Build history of the part. All positions in model axes, mm. A direction names the side the tool comes from. Give positions to 0.01 mm unless a question says otherwise; leave off trailing zeros. Loops run counter-clockwise (first coordinate to the right, second up) from the corner with the lowest first, then second, coordinate; pieces in that order, holes last. Notation, with made-up numbers: M 67.5,5.25 L 99.5,5.25 A17 ccw 99.5,18.25 Z; hole C 74.25,-19 d11. An arc over 180 degrees is marked long. Answer in a Markdown table with one row per item. Add a question column.
```python
from build123d import *

# Parameters (mm, degrees)
BOSS_EXTRUDE1_DEPTH = 1.5875


with BuildPart() as part:
    # Sketch1 → Boss-Extrude1 (new body)
    with BuildSketch(Plane(origin=(0, 0, 0), x_dir=(1, 0, 0), z_dir=(0, 1, 0))):
        with BuildLine():
            Line((-1.159549536, 2.070936998), (-3.090908521, 3.791368499))
            ThreePointArc((-3.090908521, 3.791368499), (-3.125119474, 3.931396235), (-3.006433754, 4.0132))
            Line((-3.006433754, 4.0132), (-1.7526, 4.0132))
            ThreePointArc((-1.7526, 4.0132), (-1.572994878, 4.087594878), (-1.4986, 4.2672))
            Line((-1.4986, 4.2672), (-1.4986, 4.7498))
            ThreePointArc((-1.4986, 4.7498), (-1.572994878, 4.929405122), (-1.7526, 5.0038))
            Line((-1.7526, 5.0038), (-4.7498, 5.0038))
            ThreePointArc((-4.7498, 5.0038), (-4.929405122, 4.929405122), (-5.0038, 4.7498))
            Line((-5.0038, 4.7498), (-5.0038, 1.7526))
            ThreePointArc((-5.0038, 1.7526), (-4.929405122, 1.572994878), (-4.7498, 1.4986))
            Line((-4.7498, 1.4986), (-4.2672, 1.4986))
            ThreePointArc((-4.2672, 1.4986), (-4.087594878, 1.572994878), (-4.0132, 1.7526))
            Line((-4.0132, 1.7526), (-4.0132, 3.006433754))
            ThreePointArc((-4.0132, 3.006433754), (-3.931396235, 3.125119474), (-3.791368499, 3.090908521))
            Line((-3.791368499, 3.090908521), (-2.070936998, 1.159549536))
            ThreePointArc((-2.070936998, 1.159549536), (-2.023228558, 1.08099247), (-2.0066, 0.9906))
            Line((-2.0066, 0.9906), (-2.0066, 0.7493))
            ThreePointArc((-2.0066, 0.7493), (-1.932205122, 0.569694878), (-1.7526, 0.4953))
            ThreePointArc((-1.7526, 0.4953), (-1.572994878, 0.420905122), (-1.4986, 0.2413))
            Line((-1.4986, 0.2413), (-1.4986, -0.2413))
            ThreePointArc((-1.4986, -0.2413), (-1.572994878, -0.420905122), (-1.7526, -0.4953))
            ThreePointArc((-1.7526, -0.4953), (-1.932205122, -0.569694878), (-2.0066, -0.7493))
            Line((-2.0066, -0.7493), (-2.0066, -0.9906))
            ThreePointArc((-2.0066, -0.9906), (-2.023228558, -1.08099247), (-2.070936998, -1.159549536))
            Line((-2.070936998, -1.159549536), (-3.791368499, -3.090908521))
            ThreePointArc((-3.791368499, -3.090908521), (-3.931396235, -3.125119474), (-4.0132, -3.006433754))
            Line((-4.0132, -3.006433754), (-4.0132, -1.7526))
            ThreePointArc((-4.0132, -1.7526), (-4.087594878, -1.572994878), (-4.2672, -1.4986))
            Line((-4.2672, -1.4986), (-4.7498, -1.4986))
            ThreePointArc((-4.7498, -1.4986), (-4.929405122, -1.572994878), (-5.0038, -1.7526))
            Line((-5.0038, -1.7526), (-5.0038, -4.7498))
            ThreePointArc((-5.0038, -4.7498), (-4.929405122, -4.929405122), (-4.7498, -5.0038))
            Line((-4.7498, -5.0038), (-1.7526, -5.0038))
            ThreePointArc((-1.7526, -5.0038), (-1.572994878, -4.929405122), (-1.4986, -4.7498))
            Line((-1.4986, -4.7498), (-1.4986, -4.2672))
            ThreePointArc((-1.4986, -4.2672), (-1.572994878, -4.087594878), (-1.7526, -4.0132))
            Line((-1.7526, -4.0132), (-3.006433754, -4.0132))
            ThreePointArc((-3.006433754, -4.0132), (-3.125119474, -3.931396235), (-3.090908521, -3.791368499))
            Line((-3.090908521, -3.791368499), (-1.159549536, -2.070936998))
            ThreePointArc((-1.159549536, -2.070936998), (-1.08099247, -2.023228558), (-0.9906, -2.0066))
            Line((-0.9906, -2.0066), (-0.7493, -2.0066))
            ThreePointArc((-0.7493, -2.0066), (-0.569694878, -1.932205122), (-0.4953, -1.7526))
            ThreePointArc((-0.4953, -1.7526), (-0.420905122, -1.572994878), (-0.2413, -1.4986))
            Line((-0.2413, -1.4986), (0.2413, -1.4986))
            ThreePointArc((0.2413, -1.4986), (0.420905122, -1.572994878), (0.4953, -1.7526))
            ThreePointArc((0.4953, -1.7526), (0.569694878, -1.932205122), (0.7493, -2.0066))
            Line((0.7493, -2.0066), (0.9906, -2.0066))
            ThreePointArc((0.9906, -2.0066), (1.08099247, -2.023228558), (1.159549536, -2.070936998))
            Line((1.159549536, -2.070936998), (3.090908521, -3.791368499))
            ThreePointArc((3.090908521, -3.791368499), (3.125119474, -3.931396235), (3.006433754, -4.0132))
            Line((3.006433754, -4.0132), (1.7526, -4.0132))
            ThreePointArc((1.7526, -4.0132), (1.572994878, -4.087594878), (1.4986, -4.2672))
            Line((1.4986, -4.2672), (1.4986, -4.7498))
            ThreePointArc((1.4986, -4.7498), (1.572994878, -4.929405122), (1.7526, -5.0038))
            Line((1.7526, -5.0038), (4.7498, -5.0038))
            ThreePointArc((4.7498, -5.0038), (4.929405122, -4.929405122), (5.0038, -4.7498))
            Line((5.0038, -4.7498), (5.0038, -1.7526))
            ThreePointArc((5.0038, -1.7526), (4.929405122, -1.572994878), (4.7498, -1.4986))
            Line((4.7498, -1.4986), (4.2672, -1.4986))
            ThreePointArc((4.2672, -1.4986), (4.087594878, -1.572994878), (4.0132, -1.7526))
            Line((4.0132, -1.7526), (4.0132, -3.006433754))
            ThreePointArc((4.0132, -3.006433754), (3.931396235, -3.125119474), (3.791368499, -3.090908521))
            Line((3.791368499, -3.090908521), (2.070936998, -1.159549536))
            ThreePointArc((2.070936998, -1.159549536), (2.023228558, -1.08099247), (2.0066, -0.9906))
            Line((2.0066, -0.9906), (2.0066, -0.7493))
            ThreePointArc((2.0066, -0.7493), (1.932205122, -0.569694878), (1.7526, -0.4953))
            ThreePointArc((1.7526, -0.4953), (1.572994878, -0.420905122), (1.4986, -0.2413))
            Line((1.4986, -0.2413), (1.4986, 0.2413))
            ThreePointArc((1.4986, 0.2413), (1.572994878, 0.420905122), (1.7526, 0.4953))
            ThreePointArc((1.7526, 0.4953), (1.932205122, 0.569694878), (2.0066, 0.7493))
            Line((2.0066, 0.7493), (2.0066, 0.9906))
            ThreePointArc((2.0066, 0.9906), (2.023228558, 1.08099247), (2.070936998, 1.159549536))
            Line((2.070936998, 1.159549536), (3.791368499, 3.090908521))
            ThreePointArc((3.791368499, 3.090908521), (3.931396235, 3.125119474), (4.0132, 3.006433754))
            Line((4.0132, 3.006433754), (4.0132, 1.7526))
            ThreePointArc((4.0132, 1.7526), (4.087594878, 1.572994878), (4.2672, 1.4986))
            Line((4.2672, 1.4986), (4.7498, 1.4986))
            ThreePointArc((4.7498, 1.4986), (4.929405122, 1.572994878), (5.0038, 1.7526))
            Line((5.0038, 1.7526), (5.0038, 4.7498))
            ThreePointArc((5.0038, 4.7498), (4.929405122, 4.929405122), (4.7498, 5.0038))
            Line((4.7498, 5.0038), (1.7526, 5.0038))
            ThreePointArc((1.7526, 5.0038), (1.572994878, 4.929405122), (1.4986, 4.7498))
            Line((1.4986, 4.7498), (1.4986, 4.2672))
            ThreePointArc((1.4986, 4.2672), (1.572994878, 4.087594878), (1.7526, 4.0132))
            Line((1.7526, 4.0132), (3.006433754, 4.0132))
            ThreePointArc((3.006433754, 4.0132), (3.125119474, 3.931396235), (3.090908521, 3.791368499))
            Line((3.090908521, 3.791368499), (1.159549536, 2.070936998))
            ThreePointArc((1.159549536, 2.070936998), (1.08099247, 2.023228558), (0.9906, 2.0066))
            Line((0.9906, 2.0066), (0.7493, 2.0066))
            ThreePointArc((0.7493, 2.0066), (0.569694878, 1.932205122), (0.4953, 1.7526))
            ThreePointArc((0.4953, 1.7526), (0.420905122, 1.572994878), (0.2413, 1.4986))
            Line((0.2413, 1.4986), (-0.2413, 1.4986))
            ThreePointArc((-0.2413, 1.4986), (-0.420905122, 1.572994878), (-0.4953, 1.7526))
            ThreePointArc((-0.4953, 1.7526), (-0.569694878, 1.932205122), (-0.7493, 2.0066))
            Line((-0.7493, 2.0066), (-0.9906, 2.0066))
            ThreePointArc((-0.9906, 2.0066), (-1.08099247, 2.023228558), (-1.159549536, 2.070936998))
        make_face()
    extrude(amount=BOSS_EXTRUDE1_DEPTH)


solid = part.part
```
(1) Wall check: line 1 (Z direction, x = -2.25, y = 0.25); line 2 (Z direction, x = -4.5, y = 0.35); line 3 (X direction, y = 1.5, z = 2.5) (3 decimals). Give the ranges that are in metal, low to high.
(2) Tool access for faces 4 (the flat face through (-4.013, 1, 2)), 5 (the flat face through (-5.004, 1, 3)): list every direction of +Z, -Z, +X, -X, +Y, -Y with a clear straight run to the whole face (end or side of a thin tool).
(3) Slice it at A-A, the plane x = -4.5. Give the cut face in (y, z).
(4) Slice it at B-B, the plane z = 4.5. Give the cut face in (x, y), then the cut area to 3 significant figures.
(5) Pull direction Z, two halves, no side cores. Call faces 1 (the flat face through (-2.92, 0.78, 2.11)), 2 (the flat face through (-3, 1, -5.004)), 3 (the flat face through (-5.004, 1, -3)): +Z half, -Z half, draft (parallel to the pull), parting line (faces both ways), or undercut.
(6) Slice it at D-D, the plane z = -2.25. Give the cut face in (x, y).
(7) Slice it at C-C, the plane x = 2.5. Give the cut face in (y, z) (1 decimal).
Solution:
| question | item | result |
|---|---|---|
| 1 | line 1 | -5 to -4.01, -3.04 to -1.36, 1.36 to 3.04, 4.01 to 5 |
| 1 | line 2 | -5 to -1.5, 1.5 to 5 |
| 1 | line 3 | -5.004 to -4.013, -3.265 to -1.641, 1.641 to 3.265, 4.013 to 5.004 |
| 2 | face 4 | +Y, -Y |
| 2 | face 5 | +Z, -Z, -X, +Y, -Y |
| 3 | outline | M 0,-5 L 1.59,-5 L 1.59,-1.5 L 0,-1.5 Z; M 0,1.5 L 1.59,1.5 L 1.59,5 L 0,5 Z |
| 4 | outline | M -5,0 L -1.5,0 L -1.5,1.59 L -5,1.59 Z; M 1.5,0 L 5,0 L 5,1.59 L 1.5,1.59 Z |
| 4 | area | 11.1 mm^2 |
| 5 | face 1 | undercut |
| 5 | face 2 | -Z half |
| 5 | face 3 | draft |
| 6 | outline | M -5,0 L -4.01,0 L -4.01,1.59 L -5,1.59 Z; M -3.04,0 L -1.36,0 L -1.36,1.59 L -3.04,1.59 Z; M 1.36,0 L 3.04,0 L 3.04,1.59 L 1.36,1.59 Z; M 4.01,0 L 5,0 L 5,1.59 L 4.01,1.59 Z |
| 7 | outline | M 0,-5 L 1.6,-5 L 1.6,-4 L 0,-4 Z; M 0,-3.3 L 1.6,-3.3 L 1.6,-1.6 L 0,-1.6 Z; M 0,1.6 L 1.6,1.6 L 1.6,3.3 L 0,3.3 Z; M 0,4 L 1.6,4 L 1.6,5 L 0,5 Z |
